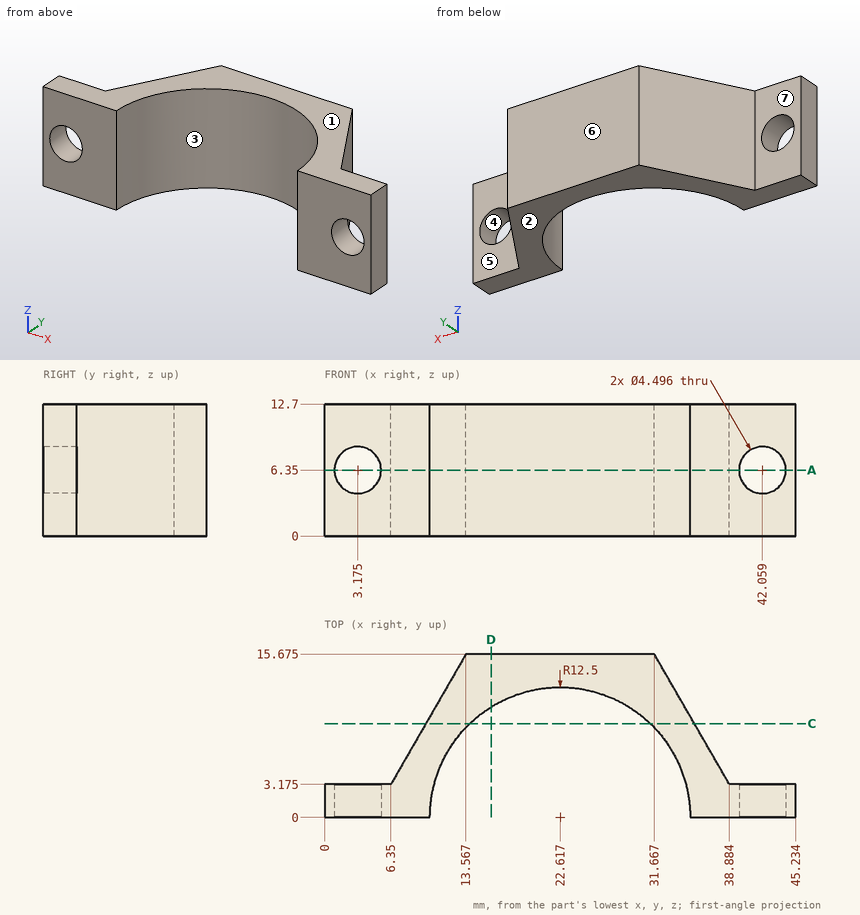
Study the drawing (mm; zero at the part's minimum x, y, z) and answer. A direction names the side the tool comes from. Coordinates: 2 decimals unless noted, no trailing zeros. Loops run counter-clockwise (first coordinate to the right, second up) from the corner with the lowest first, then second, coordinate; pieces in that order, holes last. Notation, with made-up numbers: (5.5, -35) -> (46.5, -35) arc R21 ccw to (46.5, -24) -> close; hole circle Ø3 at (-15.5, 34). An arc over 180 degrees is marked (long way). Write each question's results on one line, items separated by ' | '. Start each with the question number.
1) Consider line 1 along X through (y, z) = (11, 9) (1 decimal); line 2 along Z through (x, y) = (43, 2.5); line 3 along X through (y, z) = (7, 4.5) (1 decimal). Determine where each line is inside the solid, lowest interval first.
2) Find section A-A on z = 6.35. Count the separate pieces of the cut face and the enclosed holes in it, then the cut area to 3 significant figures.
3) Flat-ended cylindrical pins translate along their axes: P1, Ø1.5, axis at y = 10, z = 2.5, coming from the +X side; P2, Ø3, axis at x = 42.5, z = 5, coming from the +Y side (3 decimals); P3, Ø3.5, axis at x = 3.175, z = 6.35, coming from the +Y side; P4, Ø1, axis at y = 10, z = 6, coming from the +X side. Find the tip coordinate at first contact, or state that the pin passes through.
4) Find section D-D on x = 16. Determine the outline of the cut face in (y, z) (1 decimal).
5) Find section C-C on y = 9. Determine the outline of the cut face in (x, z), then the cut area to 3 significant figures.
6) The mould has two halves that part along Z. Classify the marked faces 1, 2, 3 and 4: pulls with the +Z half, pulls with the -Z half, needs draft (parallel to the pull), parting line crosses it, or undercut.
7) For the marked faces 5, 6 and 7, determine the directions among +Z, -Z, +X, -X, +Y, -Y from which every point of the face is accessible in a straight line to the end or side of a thin tool.
Response values:
1) line 1: x = 10.9 to 16.7, 28.6 to 34.4 | line 2: z = 0 to 4.31, 8.39 to 12.7 | line 3: x = 8.6 to 12.3, 33 to 36.7
2) separate pieces: 3 | enclosed holes: 0 | area: 186 mm^2
3) P1: stops at x = 35.38 | P2: stops at y = 3.175 | P3: passes through | P4: stops at x = 35.23
4) outline: (10.6, 0) -> (15.7, 0) -> (15.7, 12.7) -> (10.6, 12.7) -> close
5) outline: (9.71, 0) -> (13.94, 0) -> (13.94, 12.7) -> (9.71, 12.7) -> close; (31.29, 0) -> (35.52, 0) -> (35.52, 12.7) -> (31.29, 12.7) -> close | area: 107 mm^2
6) face 1: pulls with the +Z half | face 2: pulls with the -Z half | face 3: needs draft | face 4: undercut
7) face 5: +Z, -Z, +X, +Y | face 6: +Z, -Z, +X, -X, +Y | face 7: +Z, -Z, -X, +Y
